Print and shaded views of the part. All mm, measured from the part's lowest x, y and z. A direction names the side the tool comes from. Coordinates: 2 decimals unless noted, no trailing zeros. Write each loop counter-clockwise with the first axis right and the second up, starting at its lowest first coordinate (ties: lowest second). Pieces come first, ordered by that corner, then holes. Notation, with made-up numbers: (77.25, 27.5) -> (132.25, 27.5) arc R33 ccw to (132.25, 66.5) -> close; hole circle Ø7 at (70.5, 40). An arc over 180 degrees is marked (long way). Write item = value, one per line.
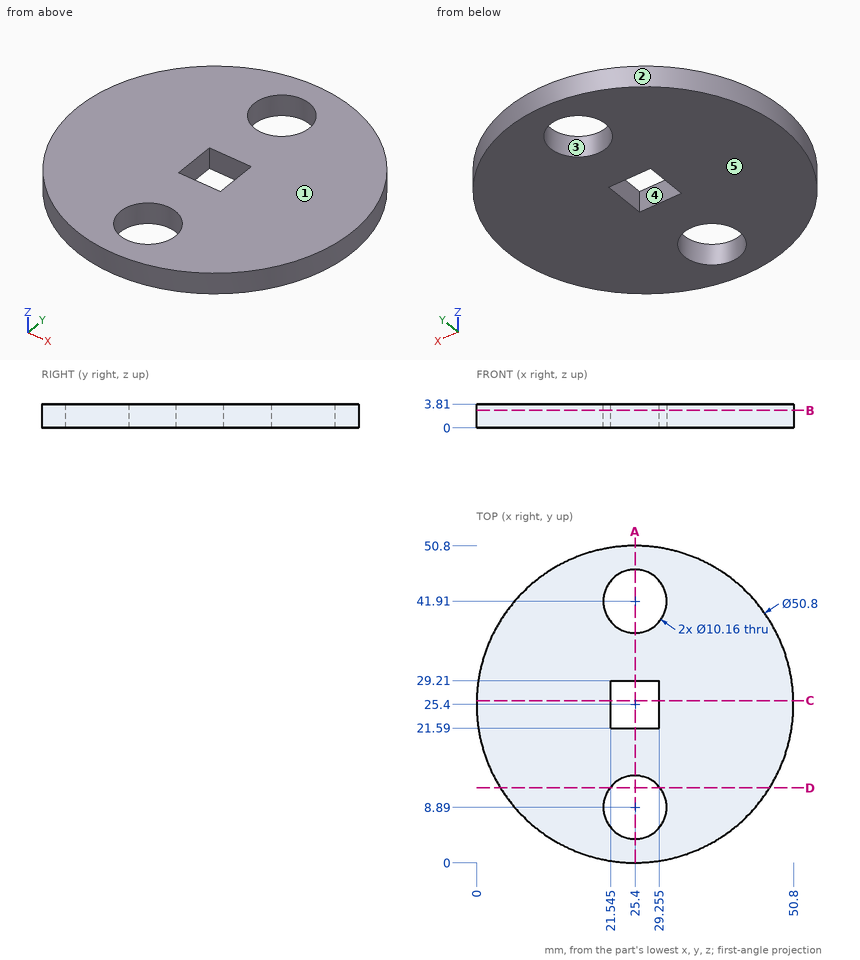
Q1. Probe line 1 (Y direction, x = 25.4, z = 2.6); line 2 (X direction, y = 26, z = 0.95) (1 decimal); line 3 (X direction, y = 39, z = 0.6) (1 decimal). List the from-to ranges inside material, lowest first. Write a range as from..to.
Model answer:
line_1 = 0..3.81, 13.97..21.59, 29.21..36.83, 46.99..50.8
line_2 = 0..21.5, 29.3..50.8
line_3 = 3.9..21.2, 29.6..46.9
Q2. Which spindle directions (+Z, -Z, +X, -X, +Y, -Y) get a long thin tool onto all of the face, cutting with end or side? Do the marked faces 4 and 5. Say none if no direction does.
Model answer:
face_4 = +Z, -Z
face_5 = -Z, +X, -X, +Y, -Y
Q3. Pin check, flat tips, straight feed: pin 1 (2 mm diameter, centred on x = 22.5, y = 42, fed in from +Z); pin 2 (1.1 mm diameter, centred on x = 27, z = 2, fed in from -Y); pin 3 (1.9 mm diameter, centred on x = 24, z = 2.5, fed in from +Y); pin 4 (1 mm diameter, centred on y = 43, z = 1.5, fed in from +X). Stop position of each tip, or through.
Model answer:
pin_1 = through
pin_2 = 0.02
pin_3 = 50.8
pin_4 = 44.18
Q4. Saw through at B-B on z = 2.8. Give the cut face in (x, y) (1 decimal).
Model answer:
outline = circle Ø50.8 at (25.4, 25.4); hole circle Ø10.2 at (25.4, 8.9); hole circle Ø10.2 at (25.4, 41.9); hole (21.5, 21.6) -> (29.3, 21.6) -> (29.3, 29.2) -> (21.5, 29.2) -> close
Q5. Mould opens along Y. For the marked faces 1, 2 and 3 say: released by +Y, released by -Y, zero draft, split by the parting line, or undercut.
Model answer:
face_1 = zero draft
face_2 = split by the parting line
face_3 = undercut
Q6. Saw through at C-C on y = 26. Give the cut face in (x, z) (1 decimal).
Model answer:
outline = (0, 0) -> (21.5, 0) -> (21.5, 3.8) -> (0, 3.8) -> close; (29.3, 0) -> (50.8, 0) -> (50.8, 3.8) -> (29.3, 3.8) -> close
Q7. Saw through at A-A on x = 25.4. Give the cut face in (y, z).
Model answer:
outline = (0, 0) -> (3.81, 0) -> (3.81, 3.81) -> (0, 3.81) -> close; (13.97, 0) -> (21.59, 0) -> (21.59, 3.81) -> (13.97, 3.81) -> close; (29.21, 0) -> (36.83, 0) -> (36.83, 3.81) -> (29.21, 3.81) -> close; (46.99, 0) -> (50.8, 0) -> (50.8, 3.81) -> (46.99, 3.81) -> close
Q8. Saw through at D-D on y = 12. Give the cut face in (x, z), and give its area (3 significant figures).
Model answer:
outline = (3.82, 0) -> (21.38, 0) -> (21.38, 3.81) -> (3.82, 3.81) -> close; (29.42, 0) -> (46.98, 0) -> (46.98, 3.81) -> (29.42, 3.81) -> close
area = 134 mm²
